Part model, mm, in its own coordinate system. A direction names the side the tool comes from. Give positions to 0.01 mm unless a question says otherwise; leave off trailing zeros. Write each loop counter-clockwise with the first axis right and the second up, starting at its lowest first coordinate (ties: lowest second). Pieces come first, ordered by that corner, then holes.
Solid Edge part; units mm, degrees
sketch "Sketch1" plane through (0, 0, 0) normal (0, -1, 0) x (1, 0, 0)
  line L0 (-7.5, -7.5) -> (7.5, -7.5)
  line L1 (7.5, -7.5) -> (7.5, 7.5)
  line L2 (7.5, 7.5) -> (-7.5, 7.5)
  line L3 (-7.5, 7.5) -> (-7.5, -7.5)
  dimension "D1" = 7.5
  dimension "D2" = 7.5
extrude "Protrusion1" add sketch "Sketch1" along normal blind 25
sketch "Sketch2" plane through (7.5, -10, 0) normal (1, 0, 0) x (0, 1, 0)
  line L0 (-15, 7.5) -> (-35, 7.5)
  line L1 (-35, 7.5) -> (-35, 0)
  line L2 (-35, 0) -> (-15, 0)
  line L3 (-15, 0) -> (-15, 7.5)
  dimension "D1" = 15
extrude "Protrusion2" add sketch "Sketch2" against normal up to vertex (15 mm away)
fillet "Verrundung_1" radius 7.5 2 edges at (7.5, -45, 3.75) (-7.5, -45, 3.75)
sketch "Sketch3" plane through (0, -17.5, 7.5) normal (0, 0, 1) x (1, 0, 0)
  circle A0 centre (0, -20) radius 2.05
extrude "Cutout1" cut sketch "Sketch3" against normal through all
chamfer "Fase_1" distance 1 angle 45 2 edges at (2.05, -37.5, 0) (-2.05, -37.5, 7.5)
chamfer "Fase_2" distance 2 angle 45 4 edges at (0, 0, 7.5) (7.5, 0, 0) (0, 0, -7.5) (-7.5, 0, 0)
1) Saw through at D-D (x = 4). Write the cut outline in (y, z).
Check result:
outline: (-43.84, 0) - (-25, 0) - (-25, -7.5) - (-2, -7.5) - (0, -5.5) - (0, 5.5) - (-2, 7.5) - (-43.84, 7.5) - close
2) 3-axis set-ups, long thin cutter, end or side, ignore diameter. For faces 5 (the flat face through (-0.1, -1, 6.5)), 6 (the flat face through (0, -33, 0)): which of +Z, -Z, +X, -X, +Y, -Y reach the whole face in a straight line?
Check result:
face 5: +Z, +X, -X, +Y
face 6: -Z, +X, -X, -Y
3) Saw through at B-B (z = -6). Write the cut outline in (x, y).
Check result:
outline: (-7.5, -25) - (7.5, -25) - (7.5, -2) - (6, -0.5) - (-6, -0.5) - (-7.5, -2) - close
4) Saw through at C-C (y = -26.5). Write the cut outline in (x, z), and give its area (4 significant figures).
Check result:
outline: (-7.5, 0) - (7.5, 0) - (7.5, 7.5) - (-7.5, 7.5) - close
area: 112.5 mm2
5) Mould opens along X. For faces 1 (the flat face through (7.5, -16, 0)), 2 (the cylindrical face through (-0.267, -35.467, 3.788)), 3 (the flat face through (0, -25, -4)), 4 (the flat face through (-6.5, -1, 0.1)) say: +X half, -X half, draft (parallel to the pull), parting line (faces both ways), or undercut.
Check result:
face 1: +X half
face 2: undercut
face 3: draft
face 4: -X half
6) Drill centre lines: L1, parallel to Y at x = 0, z = 5.2; L2, parallel to Z at x = -4, y = -41; L3, parallel to Y at x = -4, z = -3. Where is each one in solid material? Low to high.
Check result:
L1: y = -45 to -39.55, -35.45 to 0
L2: z = 0 to 7.5
L3: y = -25 to 0
7) Flat gauge pins, fed straight in: P1, Ø1, axis at y = -39, z = 4, coming from the +X side; P2, Ø4.5, axis at x = 3, y = -36.5, coming from the -Z side. Where does each tip first touch, or does it go through?
Check result:
P1: stops at x = 7.43
P2: stops at z = 0
